from build123d import *

# Parameters (mm, degrees)
SKETCH_W            = 152.4
SKETCH_H            = 63.5
PAD_DEPTH           = 25.4
FILLET_R            = 1.27
SKETCH001_W         = 146.05
SKETCH001_H         = 57.15
POCKET_DEPTH        = 22.225
SKETCH002_R         = 14.986
POCKET001_DEPTH     = 12.7
SKETCH010_R         = 3.683
PAD002_DEPTH        = 15.1384
SKETCH011_R         = 4.052374
PAD003_DEPTH        = 10.7696
SKETCH012_R         = 1.524
HOLE_DEPTH          = 8.382
HOLE_TIPS_R         = 1.524
SKETCH013_R         = 1.524
HOLE004_DEPTH       = 12.7
HOLE004_TIPS_R      = 1.524
SKETCH014_R         = 3.81
PAD004_DEPTH        = 6.985
HOLE005_D           = 3.4
HOLE005_DEPTH       = 75.7936
HOLE005_CSINK_D     = 6.7056
HOLE005_CSINK_ANGLE = 90
SKETCH016_R         = 7.62
POCKET002_DEPTH     = 5.0038
SKETCH017_R         = 3.81
PAD005_DEPTH        = 6.985
HOLE006_D           = 3.4
HOLE006_DEPTH       = 24.9936
HOLE006_CSINK_D     = 6.7
HOLE006_CSINK_ANGLE = 90
HOLE006_TIPS_R      = 1.7
SKETCH019_R         = 4.445
PAD006_DEPTH        = 3.175
SKETCH020_R         = 2.667
HOLE007_DEPTH       = 12.7
HOLE007_TIPS_R      = 2.667
SKETCH021_R         = 4.445
PAD007_DEPTH        = 3.175
SKETCH022_R         = 2.667
HOLE008_DEPTH       = 12.7
HOLE008_TIPS_R      = 2.667
HOLE009_D           = 2.9
HOLE009_DEPTH       = 24.9936
HOLE009_CSINK_D     = 6.1
HOLE009_CSINK_ANGLE = 90
HOLE009_TIPS_R      = 1.45


with BuildPart() as part:
    # Sketch → Pad (new body)
    with BuildSketch(Plane.XY):
        Rectangle(SKETCH_W, SKETCH_H)
    extrude(amount=PAD_DEPTH)

    # Fillet
    fillet_edges = [part.edges().sort_by_distance(p)[0] for p in [
        (76.2, -31.75, 12.7),
        (76.2, 31.75, 12.7),
        (-76.2, 31.75, 12.7),
        (-76.2, -31.75, 12.7),
    ]]
    fillet(fillet_edges, radius=FILLET_R)

    # Sketch001 (on Face5 of Fillet) → Pocket (cut)
    with BuildSketch(Plane.XY.offset(25.4)):
        Rectangle(SKETCH001_W, SKETCH001_H)
    extrude(amount=-POCKET_DEPTH, mode=Mode.SUBTRACT)

    # Sketch002 (on Face10 of Pocket) → Pocket001 (cut)
    with BuildSketch(Plane.YZ.offset(76.2)):
        with Locations((-3.175, 25.273)):
            Circle(SKETCH002_R)
    extrude(amount=-POCKET001_DEPTH, mode=Mode.SUBTRACT)

    # Sketch010 → Pad002 (join)
    with BuildSketch(Plane.XY.offset(3.175)):
        with Locations((-21.209, -16.1036)):
            Circle(SKETCH010_R)
        with Locations((36.195, -16.1036)):
            Circle(SKETCH010_R)
        with Locations((-21.209, 7.1374)):
            Circle(SKETCH010_R)
    extrude(amount=PAD002_DEPTH)

    # Sketch011 (on Face16 of Pad002) → Pad003 (join)
    with BuildSketch(Plane.XY.offset(3.175)):
        with Locations((36.195, 7.1374)):
            Circle(SKETCH011_R)
    extrude(amount=PAD003_DEPTH)

    # Sketch012 (on Face24 of Pad003) → Hole (cut)
    with BuildSketch(Plane.XY.offset(13.9446)):
        with Locations((36.195, 7.1374)):
            Circle(SKETCH012_R)
    extrude(amount=-HOLE_DEPTH, mode=Mode.SUBTRACT)

    # Hole tips → Hole tip 1 section 0
    with BuildSketch(Plane.XY.offset(5.5626), mode=Mode.PRIVATE) as hole_tip_1_s0:
        with Locations((36.195, 7.1374)):
            Circle(HOLE_TIPS_R)
    loft([hole_tip_1_s0.sketch, Vertex(36.195, 7.1374, 4.646888)], mode=Mode.SUBTRACT)

    # Sketch013 (on Face23 of Hole) → Hole004 (cut)
    with BuildSketch(Plane.XY.offset(18.3134)):
        with Locations((-21.209, 7.1374)):
            Circle(SKETCH013_R)
        with Locations((36.195, -16.1036)):
            Circle(SKETCH013_R)
        with Locations((-21.209, -16.1036)):
            Circle(SKETCH013_R)
    extrude(amount=-HOLE004_DEPTH, mode=Mode.SUBTRACT)

    # Hole004 tips → Hole004 tip 1 section 0
    with BuildSketch(Plane.XY.offset(5.6134), mode=Mode.PRIVATE) as hole004_tip_1_s0:
        with Locations((-21.209, 7.1374)):
            Circle(HOLE004_TIPS_R)
    loft([hole004_tip_1_s0.sketch, Vertex(-21.209, 7.1374, 4.697688)], mode=Mode.SUBTRACT)

    # Hole004 tips → Hole004 tip 2 section 0
    with BuildSketch(Plane.XY.offset(5.6134), mode=Mode.PRIVATE) as hole004_tip_2_s0:
        with Locations((36.195, -16.1036)):
            Circle(HOLE004_TIPS_R)
    loft([hole004_tip_2_s0.sketch, Vertex(36.195, -16.1036, 4.697688)], mode=Mode.SUBTRACT)

    # Hole004 tips → Hole004 tip 3 section 0
    with BuildSketch(Plane.XY.offset(5.6134), mode=Mode.PRIVATE) as hole004_tip_3_s0:
        with Locations((-21.209, -16.1036)):
            Circle(HOLE004_TIPS_R)
    loft([hole004_tip_3_s0.sketch, Vertex(-21.209, -16.1036, 4.697688)], mode=Mode.SUBTRACT)

    # Sketch014 (on Face16 of Hole004) → Pad004 (join)
    with BuildSketch(Plane.XY.offset(3.175)):
        with Locations((-68.3768, 24.13)):
            Circle(SKETCH014_R)
        with Locations((-68.3768, -24.13)):
            Circle(SKETCH014_R)
    extrude(amount=PAD004_DEPTH)

    # Hole005
    with Locations(Plane(origin=(0, 0, 0), x_dir=(1, 0, 0), z_dir=(0, 0, -1))):
        with Locations((-68.58, 24.13), (-68.58, -24.13)):
            CounterSinkHole(HOLE005_D / 2, HOLE005_CSINK_D / 2, depth=HOLE005_DEPTH, counter_sink_angle=HOLE005_CSINK_ANGLE)

    # Sketch016 (on Face1 of Hole005) → Pocket002 (cut)
    with BuildSketch(Plane(origin=(-76.2, 0, 0), x_dir=(0, -1, 0), z_dir=(-1, 0, 0))):
        with Locations((0, 12.7)):
            Circle(SKETCH016_R)
    extrude(amount=-POCKET002_DEPTH, mode=Mode.SUBTRACT)

    # Sketch017 (on Face21 of Pocket002) → Pad005 (join)
    with BuildSketch(Plane.XY.offset(3.175)):
        with Locations((47.625, -23.368)):
            Circle(SKETCH017_R)
        with Locations((47.625, 23.368)):
            Circle(SKETCH017_R)
    extrude(amount=PAD005_DEPTH)

    # Hole006
    with Locations(Plane(origin=(0, 0, 0), x_dir=(1, 0, 0), z_dir=(0, 0, -1))):
        with Locations((47.625, 23.368), (47.625, -23.368)):
            CounterSinkHole(HOLE006_D / 2, HOLE006_CSINK_D / 2, depth=HOLE006_DEPTH, counter_sink_angle=HOLE006_CSINK_ANGLE)

    # Hole006 tips → Hole006 tip 1 section 0
    with BuildSketch(Plane(origin=(0, 0, 24.9936), x_dir=(1, 0, 0), z_dir=(0, 0, -1)), mode=Mode.PRIVATE) as hole006_tip_1_s0:
        with Locations((47.625, 23.368)):
            Circle(HOLE006_TIPS_R)
    loft([hole006_tip_1_s0.sketch, Vertex(47.625, -23.368, 26.015063)], mode=Mode.SUBTRACT)

    # Hole006 tips → Hole006 tip 2 section 0
    with BuildSketch(Plane(origin=(0, 0, 24.9936), x_dir=(1, 0, 0), z_dir=(0, 0, -1)), mode=Mode.PRIVATE) as hole006_tip_2_s0:
        with Locations((47.625, -23.368)):
            Circle(HOLE006_TIPS_R)
    loft([hole006_tip_2_s0.sketch, Vertex(47.625, 23.368, 26.015063)], mode=Mode.SUBTRACT)

    # Sketch019 (on Face20 of Hole006) → Pad006 (join)
    with BuildSketch(Plane(origin=(0, -28.575, 0), x_dir=(-1, 0, 0), z_dir=(0, 1, 0))):
        with Locations((-41.275, 15.875)):
            Circle(SKETCH019_R)
        with Locations((41.275, 15.875)):
            Circle(SKETCH019_R)
    extrude(amount=PAD006_DEPTH)

    # Sketch020 (on Face8 of Pad006) → Hole007 (cut)
    with BuildSketch(Plane.XZ.offset(31.75)):
        with Locations((-41.275, 15.875)):
            Circle(SKETCH020_R)
        with Locations((41.275, 15.875)):
            Circle(SKETCH020_R)
    extrude(amount=-HOLE007_DEPTH, mode=Mode.SUBTRACT)

    # Hole007 tips → Hole007 tip 1 section 0
    with BuildSketch(Plane.XZ.offset(19.05), mode=Mode.PRIVATE) as hole007_tip_1_s0:
        with Locations((-41.275, 15.875)):
            Circle(HOLE007_TIPS_R)
    loft([hole007_tip_1_s0.sketch, Vertex(-41.275, -17.447505, 15.875)], mode=Mode.SUBTRACT)

    # Hole007 tips → Hole007 tip 2 section 0
    with BuildSketch(Plane.XZ.offset(19.05), mode=Mode.PRIVATE) as hole007_tip_2_s0:
        with Locations((41.275, 15.875)):
            Circle(HOLE007_TIPS_R)
    loft([hole007_tip_2_s0.sketch, Vertex(41.275, -17.447505, 15.875)], mode=Mode.SUBTRACT)

    # Sketch021 (on Face18 of Hole007) → Pad007 (join)
    with BuildSketch(Plane.XZ.offset(-28.575)):
        with Locations((-41.275, 15.875)):
            Circle(SKETCH021_R)
        with Locations((41.275, 15.875)):
            Circle(SKETCH021_R)
    extrude(amount=PAD007_DEPTH)

    # Sketch022 (on Face7 of Pad007) → Hole008 (cut)
    with BuildSketch(Plane(origin=(0, 31.75, 0), x_dir=(-1, 0, 0), z_dir=(0, 1, 0))):
        with Locations((-41.275, 15.875)):
            Circle(SKETCH022_R)
        with Locations((41.275, 15.875)):
            Circle(SKETCH022_R)
    extrude(amount=-HOLE008_DEPTH, mode=Mode.SUBTRACT)

    # Hole008 tips → Hole008 tip 1 section 0
    with BuildSketch(Plane(origin=(0, 19.05, 0), x_dir=(-1, 0, 0), z_dir=(0, 1, 0)), mode=Mode.PRIVATE) as hole008_tip_1_s0:
        with Locations((-41.275, 15.875)):
            Circle(HOLE008_TIPS_R)
    loft([hole008_tip_1_s0.sketch, Vertex(41.275, 17.447505, 15.875)], mode=Mode.SUBTRACT)

    # Hole008 tips → Hole008 tip 2 section 0
    with BuildSketch(Plane(origin=(0, 19.05, 0), x_dir=(-1, 0, 0), z_dir=(0, 1, 0)), mode=Mode.PRIVATE) as hole008_tip_2_s0:
        with Locations((41.275, 15.875)):
            Circle(HOLE008_TIPS_R)
    loft([hole008_tip_2_s0.sketch, Vertex(-41.275, 17.447505, 15.875)], mode=Mode.SUBTRACT)

    # Hole009
    with Locations(Plane.YZ.offset(76.2)):
        with Locations((-17.653, 10.922), (11.303, 10.922)):
            CounterSinkHole(HOLE009_D / 2, HOLE009_CSINK_D / 2, depth=HOLE009_DEPTH, counter_sink_angle=HOLE009_CSINK_ANGLE)

    # Hole009 tips → Hole009 tip 1 section 0
    with BuildSketch(Plane.YZ.offset(51.2064), mode=Mode.PRIVATE) as hole009_tip_1_s0:
        with Locations((-17.653, 10.922)):
            Circle(HOLE009_TIPS_R)
    loft([hole009_tip_1_s0.sketch, Vertex(50.335152, -17.653, 10.922)], mode=Mode.SUBTRACT)

    # Hole009 tips → Hole009 tip 2 section 0
    with BuildSketch(Plane.YZ.offset(51.2064), mode=Mode.PRIVATE) as hole009_tip_2_s0:
        with Locations((11.303, 10.922)):
            Circle(HOLE009_TIPS_R)
    loft([hole009_tip_2_s0.sketch, Vertex(50.335152, 11.303, 10.922)], mode=Mode.SUBTRACT)


solid = part.part
The model under review builds one solid part; all positions refer to its coordinate system, in mm. A direction names the side the tool comes from. Give positions to 0.01 mm unless a question says otherwise; leave off trailing zeros. Order: outer loops, then holes, each group sorted by start corner. A loop starts at its lowest first (then second) coordinate and runs counter-clockwise, first axis right, second up. Notation, with made-up numbers: M 84,-20.75 L 118,-20.75 A12 ccw 118,-0.75 Z; hole C 50,-33.5 d3. An arc over 180 degrees is marked long. Answer in a Markdown table with one row per item. Add a question column.
1. To check wall thickness, follow line 1 along Y through (x, z) = (-68.58, 4.5) (3 decimals); line 2 along X through (y, z) = (29.5, 16); line 3 along Y through (x, z) = (6.5, 14) (3 decimals). State the ranges of each line that lie inside material, in increasing order.
2. Mouldability with a two-part tool opening along Z and no side actions: class faces 1 (the cylindrical face through (-71.4, 21.81, 6.62)), 2 (the cylindrical face through (-45.515, -27.01, 17.21)), 3 (the flat face through (-66.7, -24.1, 10.16)) as released by +Z, released by -Z, zero draft, split by the parting line, or undercut.
3. Machinability: for faces 4 (the cylindrical face through (-74.635, 0.992, 20.255)), 5 (the cylindrical face through (73.8, 12.75, 10.99)), 6 (the cylindrical face through (43.39, 28.62, 14.25)), 7 (the cylindrical face through (34.672, -16.037, 12.052)), 8 (the cylindrical face through (37.035, -27.01, 17.21)), which of the approach directions +Z, -Z, +X, -X, +Y, -Y give a long, thin tool a straight path to every point of the face, cutting with its end or side? Answer none if there is none.
4. Add section B-B on x = -68.58. State the section outline as (y, z) points (3 decimals).
5. Add section A-A on y = 0. State the section outline as (x, z) points (3 decimals).
6. Add section C-C on x = -15. State the section outline as (y, z) points (3 decimals).
7. For pin 1 Ø2.5 at (x, z) = (40, 18) entering from +Y; pin 2 Ø4 at (x, y) = (-21.21, -16.1) entering from +Z; pin 3 Ø2.5 at (x, y) = (47.625, 23.368) entering from +Z; pin 4 Ø4 at (x, y) = (-67.5, 24) entering from +Z, all flat-tipped, find the tip position at first contact; note any pin that passes through.
The answers:
| question | item | result |
|---|---|---|
| 1 | line 1 | -31.75 to -28.575, -27.935 to -25.83, -22.43 to -20.325, 20.325 to 22.43, 25.83 to 27.935, 28.575 to 31.75 |
| 1 | line 2 | -76.2 to -43.94, -38.61 to 38.61, 43.94 to 76.2 |
| 1 | line 3 | -31.75 to -28.575, 28.575 to 31.75 |
| 2 | face 1 | zero draft |
| 2 | face 2 | undercut |
| 2 | face 3 | released by +Z |
| 3 | face 4 | -X |
| 3 | face 5 | +X |
| 3 | face 6 | +Y |
| 3 | face 7 | +Z |
| 3 | face 8 | none |
| 4 | outline | M -31.75,0 L -27.483,0 L -25.83,1.653 L -25.83,10.16 L -27.935,10.16 L -27.935,3.175 L -28.575,3.175 L -28.575,25.4 L -31.75,25.4 Z; M -22.43,1.653 L -20.777,0 L 20.777,0 L 22.43,1.653 L 22.43,10.16 L 20.325,10.16 L 20.325,3.175 L -20.325,3.175 L -20.325,10.16 L -22.43,10.16 Z; M 25.83,1.653 L 27.483,0 L 31.75,0 L 31.75,25.4 L 28.575,25.4 L 28.575,3.175 L 27.935,3.175 L 27.935,10.16 L 25.83,10.16 Z |
| 5 | outline | M -76.2,0 L 76.2,0 L 76.2,10.627 L 73.025,10.627 L 73.025,3.175 L -73.025,3.175 L -73.025,5.08 L -76.2,5.08 Z; M -76.2,20.32 L -73.025,20.32 L -73.025,25.4 L -76.2,25.4 Z |
| 6 | outline | M -31.75,0 L 31.75,0 L 31.75,25.4 L 28.575,25.4 L 28.575,3.175 L -28.575,3.175 L -28.575,25.4 L -31.75,25.4 Z |
| 7 | pin 1 | y = 31.75 |
| 7 | pin 2 | z = 18.31 |
| 7 | pin 3 | through |
| 7 | pin 4 | z = 10.16 |
